from build123d import *
from build123d.topology import SkipClean

# Parameters (mm, degrees)
SKETCH1_R           = 3.45
BOSS_EXTRUDE1_DEPTH = 1.1
SKETCH2_R           = 6.7
BOSS_EXTRUDE2_DEPTH = 4.3
SKETCH3_W           = 5.1
SKETCH3_H           = 2.5
CUT_EXTRUDE1_DEPTH  = 11.905961672
BOSS_EXTRUDE3_START = 4
BOSS_EXTRUDE3_DEPTH = 4
CHAMFER1_SIZE       = 0.8
BOSS_EXTRUDE4_DEPTH = 3.6


with BuildPart() as part:
    # Sketch1 → Boss-Extrude1 (new body)
    with BuildSketch(Plane(origin=(0, 0, 0), x_dir=(1, 0, 0), z_dir=(0, 1, 0))):
        with Locations(Location((0, 0, 0), (0, 0, 270))):
            Circle(SKETCH1_R)
    extrude(amount=BOSS_EXTRUDE1_DEPTH)

    # Sketch2 → Boss-Extrude2 (add)
    with BuildSketch(Plane(origin=(0, 1.1, 0), x_dir=(1, 0, 0), z_dir=(0, 1, 0))):
        with Locations(Location((0, 0, 0), (0, 0, 90))):
            Circle(SKETCH2_R)
    extrude(amount=BOSS_EXTRUDE2_DEPTH)

    # Sketch3 → Cut-Extrude1 (cut, through all)
    with BuildSketch(Plane(origin=(0, 5.4, 0), x_dir=(1, 0, 0), z_dir=(0, 1, 0))):
        Rectangle(SKETCH3_W, SKETCH3_H)
    extrude(amount=-CUT_EXTRUDE1_DEPTH, mode=Mode.SUBTRACT)

    # Sketch4 → Boss-Extrude3 (add)
    with SkipClean():  # the faces are left unmerged after this step: merging them gives an invalid solid
        with BuildSketch(Plane.XZ.offset(-1.1).offset(BOSS_EXTRUDE3_START)):
            with BuildLine():
                ThreePointArc((2.5, 6.216108107), (0, 6.7), (-2.5, 6.216108107))
                Line((-2.5, 6.216108107), (-2.5, 3.979949748))
                ThreePointArc((-2.5, 3.979949748), (0, 4.7), (2.5, 3.979949748))
                Line((2.5, 3.979949748), (2.5, 6.216108107))
            make_face()
        extrude(amount=-BOSS_EXTRUDE3_DEPTH)

    # Chamfer1
    chamfer1_edges = [part.edges().sort_by_distance(p)[0] for p in [
        (-2.5, -2.9, 5.098028928),
        (2.5, -2.9, 5.098028928),
    ]]
    chamfer(chamfer1_edges, length=CHAMFER1_SIZE)

    # Sketch5 → Boss-Extrude4 (add)
    with SkipClean():  # the faces are left unmerged after this step: merging them gives an invalid solid
        with BuildSketch(Plane(origin=(0, 5.4, 0), x_dir=(1, 0, 0), z_dir=(0, 1, 0))):
            with BuildLine():
                Line((-2.55, -1.25), (-2.55, 1.25))
                Line((-2.55, 1.25), (2.55, 1.25))
                Line((2.55, 1.25), (2.55, -1.25))
                Line((2.55, -1.25), (2.55, -6.195764682))
                ThreePointArc((2.55, -6.195764682), (5.566641717, -3.728605638), (6.7, 0))
                ThreePointArc((6.7, 0), (-3.728605638, 5.566641717), (-2.55, -6.195764682))
                Line((-2.55, -6.195764682), (-2.55, -1.25))
            make_face()
        extrude(amount=BOSS_EXTRUDE4_DEPTH)


solid = part.part
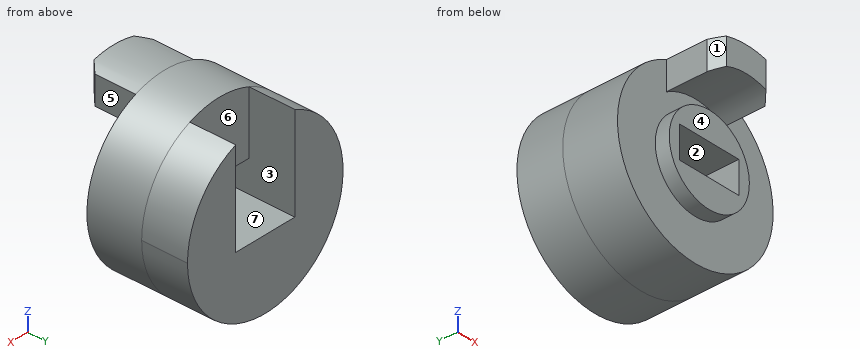
Model file for the job. Use its own axes, mm. Face numbers are marked on the shaded views. A direction names the side the tool comes from. Give positions to 0.01 mm unless a question says otherwise; leave off trailing zeros. Order: outer loops, then holes, each group sorted by start corner. A loop starts at its lowest first (then second) coordinate and runs counter-clockwise, first axis right, second up. Notation, with made-up numbers: M 69,17.25 L 96,17.25 A9 ccw 96,30.25 Z; hole C -11,33 d11. An arc over 180 degrees is marked long. Write item = value, one per line.
Q1. Cut at D-D, the plane z = -2.5. List the corners of the cut face in (x, y).
Derived:
outline = M -6.22,1.1 L -2.38,1.1 L -2.38,0 L 2.38,0 L 2.38,1.1 L 6.22,1.1 L 6.22,9 L -6.22,9 Z
Q2. Cut at A-A, the plane x = 0. List the corners of the cut face in (y, z).
Derived:
outline = M -2.9,4.7 L 1.1,4.7 L 1.1,3.45 L 0,3.45 L 0,1.25 L 5.4,1.25 L 5.4,6.7 L -2.9,6.7 Z; M 0,-3.45 L 1.1,-3.45 L 1.1,-6.7 L 9,-6.7 L 9,-1.25 L 0,-1.25 Z
Q3. Flat gauge pins, fed straight in: pin 1 (3.5 mm diameter, centred on x = 0.5, z = -1, fed in from -Y); pin 2 (4 mm diameter, centred on x = -4.5, z = -4, fed in from -Y); pin 3 (1.1 mm diameter, centred on y = 0, z = 5.5, fed in from -X). Where does each tip first touch, or does it go through?
Derived:
pin_1 = 0
pin_2 = 1.1
pin_3 = -2.5
Q4. Drill centre lines: line 1 (X direction, y = 3, z = 0); line 2 (Y direction, x = 1.5, z = 6); line 3 (Y direction, x = 0.75, z = -1.75). Where is each one in solid material? Low to high. Write a range as [from, to].
Derived:
line_1 = [-6.7, -2.55], [2.55, 6.7]
line_2 = [-2.9, 5.4]
line_3 = [0, 9]
Q5. Cut at B-B, the plane y = 2.5. List the corners of the cut face in (x, z).
Derived:
outline = C 0,0 d13.4; hole M -2.55,-1.25 L 2.55,-1.25 L 2.55,1.25 L -2.55,1.25 Z
Q6. Tool access for the marked faces 3, 4, 5, 6 and 7: list every direction of +Z, -Z, +X, -X, +Y, -Y with a clear straight run to the whole face (end or side of a thin tool).
Derived:
face_3 = +Y
face_4 = -Z, +X, -X, -Y
face_5 = +Z, +X, -Y
face_6 = +Z, +Y
face_7 = +Y, -Y
Q7. Cut at C-C, the plane y = 6. List the corners of the cut face in (x, z), then the cut area to 3 significant figures.
Derived:
outline = M -2.55,-1.25 L -2.55,6.2 A6.7 ccw long 2.55,6.2 L 2.55,-1.25 Z
area = 101 mm2
Q8. Two-plate mould, pull along Z, no slides. Class the marked faces 1 and 2: pulls with the +Z half, pulls with the -Z half, needs draft (parallel to the pull), parting line crosses it, or undercut.
Derived:
face_1 = needs draft
face_2 = undercut
